Work out the finished part from the listing and answer in its coordinate system (mm). Face numbers are marked on the shaded views. Round coordinates to 2 decimals unless told otherwise and drop trailing zeros. Write each loop counter-clockwise with the first axis right and the second up, starting at its lowest first coordinate (ties: lowest second). Pieces come first, ordered by that corner, then holes.
1. Find section A-A (z = 0). Write down the section's boundary in (x, y).
2. Find section C-C (y = 13.25). Write down the section's boundary in (x, z).
3. Flat-ended cylindrical pins translate along their axes: pin 1 Ø3 at (y, z) = (12.5, 11.5) entering from +X; pin 2 Ø5 at (y, z) = (14.5, 14.5) entering from +X; pin 3 Ø3 at (y, z) = (6, 9) entering from +X; pin 4 Ø2 at (x, z) = (-1, -0.5) entering from +Y. Find the tip coordinate at first contact, or state that the pin passes through.
4. Straight lines are drawn through the part: probe 1 along Z at (x, y) = (-6.5, 1.5); probe 2 along X at (y, z) = (16.5, -0.5); probe 3 along X at (y, z) = (6.5, 3). For each, find the intervals that lie inside material, in ascending order.
5. Determine the mould class of the marked faces 1, 2 and 3 for opening direction Z: pulls with the +Z half, pulls with the -Z half, needs draft (parallel to the pull), parting line crosses it, or undercut.
6. Find section B-B (x = -12). Write down the section's boundary in (y, z).
7. Find section D-D (z = -7). Write down the section's boundary in (x, y) (3 decimals).
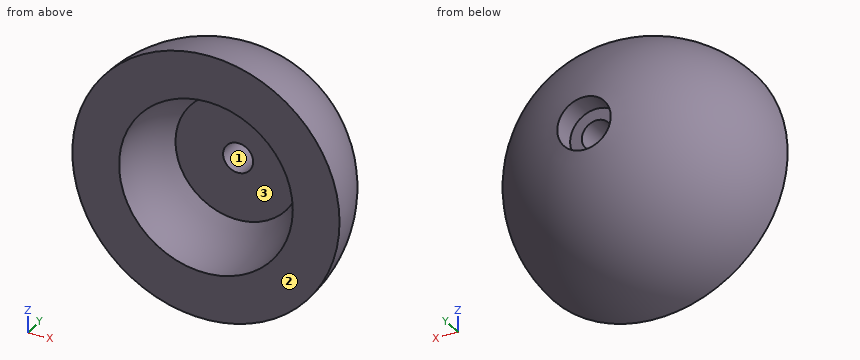
Autodesk Inventor part; units mm, degrees
ref_plane "Work Plane1" through (0, 20, 0) normal (0, 1, 0) x (-1, 0, 0)
ref_plane "YZ Plane" through (0, 0, 0) normal (1, 0, 0) x (0, 1, 0)
ref_plane "XY Plane" through (0, 0, 0) normal (0, 0, 1) x (1, 0, 0)
sketch "Sketch1" plane through (0, 0, 0) normal (0, 0, 1) x (1, 0, 0)
  line L0 (0, 0) -> (0, 20)
  line L1 (0, 0) -> (20, 0)
  arc A0 (20, 0) -> (0, 20) centre (0, 0) ccw
  line L2 (0, -4.8284) -> (0, 28.9706)
  dimension "d2" = 20
revolve "Revolution1" add sketch "Sketch1" angle 360 about axis through (0, -10, 0) along (0, 1, 0)
ref_plane "Work Plane1" through (0, 20, 0) normal (0, 1, 0) x (-1, 0, 0)
sketch "Sketch2" plane through (0, 20, 0) normal (0, 1, 0) x (-1, 0, 0)
  point P0 (0, 0)
  point P1 (0, 0)
hole "Hole1" at (0, 20, 0) direction (0, -1, 0) diameter 4.5 end through all counterbore diameter 8 counterbore depth 4
shell "Shell1" thickness 7 removed faces 1 at (13.8841, 0, 1.6858)
sketch "Sketch3" plane through (0, 0, 0) normal (0, -1, 0) x (1, 0, 0)
  circle A0 centre (0, 0) radius 9.25
  circle A1 centre (0, 0) radius 2.25
extrude "Extrusion1" cut sketch "Sketch3" against normal up to surface (9 mm away)
properties part number "Ball_Upper Half" material "Nylon 6/6"
Worked answers:
1. outline: (-20, 0) - (-13, 0) arc R13 cw to (-9.38, 9) - (-2.25, 9) - (-2.25, 16) - (-4, 16) - (-4, 19.6) arc R20 ccw to start; (2.25, 9) - (9.38, 9) arc R13 cw to (13, 0) - (20, 0) arc R20 ccw to (4, 19.6) - (4, 16) - (2.25, 16) - close
2. outline: circle Ø29.96 at (0, 0); hole circle Ø4.5 at (0, 0)
3. pin 1: stops at x = 12.66
3. pin 2: stops at x = 8.71
3. pin 3: stops at x = 17.7
3. pin 4: passes through
4. probe 1: z = -18.85 to -11.16, 11.16 to 18.85
4. probe 2: x = -11.29 to -3.97, 3.97 to 11.29
4. probe 3: x = -18.67 to -10.85, 10.85 to 18.67
5. face 1: undercut
5. face 2: needs draft
5. face 3: undercut
6. outline: (0, -16) arc R16 ccw to (0, 16) - (0, 5) arc R5 cw to (0, -5) - close
7. outline: (-18.735, 0) - (-10.954, 0) arc R10.954 cw to (-6.245, 9) - (6.245, 9) arc R10.954 cw to (10.954, 0) - (18.735, 0) arc R18.735 ccw to start
